from build123d import *

# Parameters (mm, degrees)
BOSS_EXTRUDE1_DEPTH              = 1.6
BOSS_EXTRUDE2_DEPTH              = 0.1
M1_6_HOLE1_FIXINGSTRUCTURE_D     = 1.8
M1_6_HOLE1_FIXINGSTRUCTURE_DEPTH = 200
M1_6_HOLE1_FIXINGSTRUCTURE_TIP   = 0.540774557


with BuildPart() as part:
    # Sketch1 → Boss-Extrude1 (new body)
    with BuildSketch(Plane.XY):
        with BuildLine():
            Line((-32, 38.5), (-32, 32.5))
            ThreePointArc((-32, 32.5), (-32.146446609, 32.146446609), (-32.5, 32))
            Line((-32.5, 32), (-38.5, 32))
            ThreePointArc((-38.5, 32), (-38.853553391, 31.853553391), (-39, 31.5))
            Line((-39, 31.5), (-39, -31.5))
            ThreePointArc((-39, -31.5), (-38.853553391, -31.853553391), (-38.5, -32))
            Line((-38.5, -32), (-32.5, -32))
            ThreePointArc((-32.5, -32), (-32.146446609, -32.146446609), (-32, -32.5))
            Line((-32, -32.5), (-32, -38.5))
            ThreePointArc((-32, -38.5), (-31.853553391, -38.853553391), (-31.5, -39))
            Line((-31.5, -39), (31.5, -39))
            ThreePointArc((31.5, -39), (31.853553391, -38.853553391), (32, -38.5))
            Line((32, -38.5), (32, -32.5))
            ThreePointArc((32, -32.5), (32.146446609, -32.146446609), (32.5, -32))
            Line((32.5, -32), (38.5, -32))
            ThreePointArc((38.5, -32), (38.853553391, -31.853553391), (39, -31.5))
            Line((39, -31.5), (39, 31.5))
            ThreePointArc((39, 31.5), (38.853553391, 31.853553391), (38.5, 32))
            Line((38.5, 32), (32.5, 32))
            ThreePointArc((32.5, 32), (32.146446609, 32.146446609), (32, 32.5))
            Line((32, 32.5), (32, 38.5))
            ThreePointArc((32, 38.5), (31.853553391, 38.853553391), (31.5, 39))
            Line((31.5, 39), (-31.5, 39))
            ThreePointArc((-31.5, 39), (-31.853553391, 38.853553391), (-32, 38.5))
        make_face()
    extrude(amount=BOSS_EXTRUDE1_DEPTH)

    # Esboço1 → Boss-Extrude2 (add)
    with BuildSketch(Plane.XY.offset(1.6)):
        with BuildLine():
            Line((-25, -30), (25, -30))
            ThreePointArc((25, -30), (28.535533906, -28.535533906), (30, -25))
            Line((30, -25), (30, 25))
            ThreePointArc((30, 25), (28.535533906, 28.535533906), (25, 30))
            Line((25, 30), (-25, 30))
            ThreePointArc((-25, 30), (-28.535533906, 28.535533906), (-30, 25))
            Line((-30, 25), (-30, -25))
            ThreePointArc((-30, -25), (-28.535533906, -28.535533906), (-25, -30))
        make_face()
    extrude(amount=BOSS_EXTRUDE2_DEPTH)

    # M1.6 Hole1-FixingStructure
    with Locations(Plane(origin=(0, 0, 0), x_dir=(-1, 0, 0), z_dir=(0, 0, -1))):
        with Locations((-29, 36), (29, 36), (-29, -36), (29, -36), (36, 29), (36, -29), (-36, -29), (-36, 29)):
            Hole(M1_6_HOLE1_FIXINGSTRUCTURE_D / 2, depth=M1_6_HOLE1_FIXINGSTRUCTURE_DEPTH)
            with Locations((0, 0, -(M1_6_HOLE1_FIXINGSTRUCTURE_DEPTH + M1_6_HOLE1_FIXINGSTRUCTURE_TIP / 2))):  # 118° drill point
                Cone(0, M1_6_HOLE1_FIXINGSTRUCTURE_D / 2, M1_6_HOLE1_FIXINGSTRUCTURE_TIP, mode=Mode.SUBTRACT)


solid = part.part
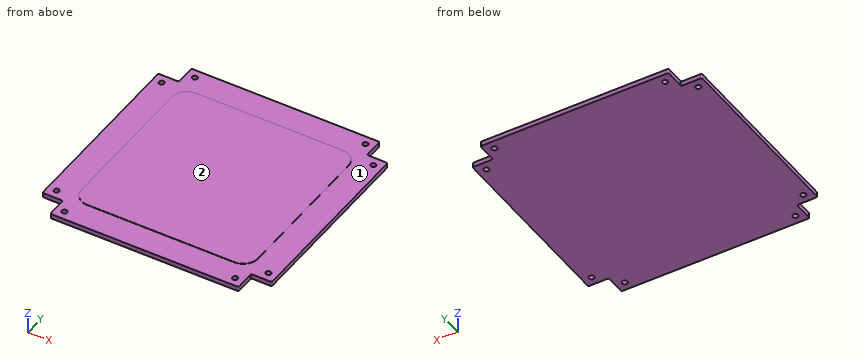
The listing builds one solid part. Answer for the finished solid, in the listing's coordinates (mm). Face numbers are marked on the shaded views. A direction names the side the tool comes from. Round coordinates to 2 decimals unless told otherwise and drop trailing zeros. Order: outer loops, then holes, each group sorted by start corner. A loop starts at its lowest first (then second) coordinate and runs counter-clockwise, first axis right, second up. Notation, with made-up numbers: (23.25, 78.25) -> (67.25, 78.25) arc R27 ccw to (67.25, 105.25) -> close; hole circle Ø10 at (20.25, 44.25). An arc over 180 degrees is marked (long way). Put each result on its own line as item: value.
Q1. Section C-C, the plane z = 1.2 is taken. Count the separate pieces of the cut face and the enclosed holes in it, and give its area (3 significant figures).
Results list:
separate pieces: 1
enclosed holes: 8
area: 5,870 mm^2
Q2. Section A-A, the plane y = 29 is taken. Write down the section's boundary in (x, z), and give its area (3 significant figures).
Results list:
outline: (-39, 0) -> (-36.9, 0) -> (-36.9, 1.6) -> (-39, 1.6) -> close; (-35.1, 0) -> (35.1, 0) -> (35.1, 1.6) -> (28, 1.6) -> (28, 1.7) -> (-28, 1.7) -> (-28, 1.6) -> (-35.1, 1.6) -> close; (36.9, 0) -> (39, 0) -> (39, 1.6) -> (36.9, 1.6) -> close
area: 125 mm^2
Q3. Which of the six approach directions +Z, -Z, +X, -X, +Y, -Y give full straight-line access (tool end or side, diameter ignored) to the marked faces 1 and 2?
Results list:
face 1: +Z
face 2: +Z, +X, -X, +Y, -Y
Q4. Each of these flat-tipped pins is pushed along its axis until it touches: P1, Ø0.5, axis at y = 34.5, z = 1, coming from the +X side; P2, Ø10, axis at x = -20, y = -31, coming from the -Z side; P3, Ø3, axis at x = -29, y = -36, coming from the +Z side. Where does it stop, or does it pass through?
Results list:
P1: x = 32
P2: z = 0
P3: z = 1.6
Q5. Consider line 1 along Y through (x, z) = (-29, 1.25); line 2 along Y through (x, z) = (36, 1.2). Determine where each line is inside the solid, lowest interval first.
Results list:
line 1: -39 to -36.9, -35.1 to 35.1, 36.9 to 39
line 2: -32 to -29.9, -28.1 to 28.1, 29.9 to 32
